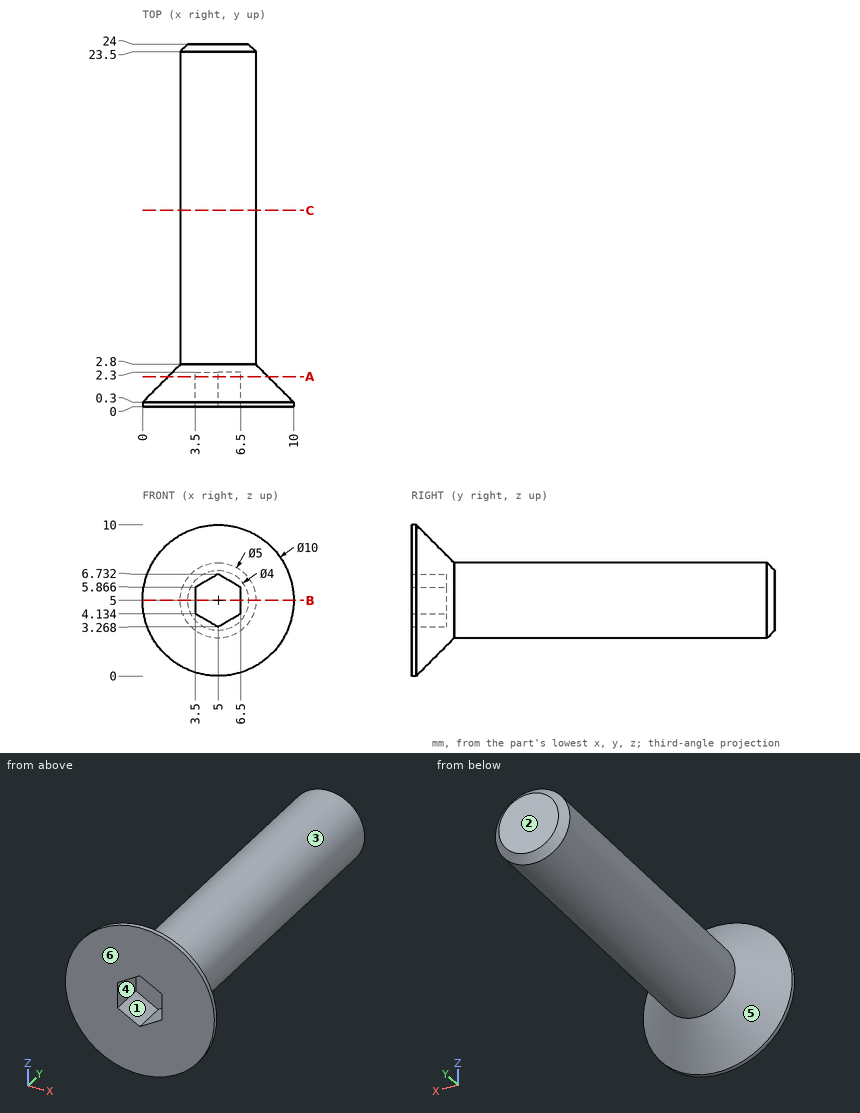
Input: dimensioned drawing with shaded views. Units: mm. Origin: part minimum x, y, z. A direction names the side the tool comes from. Coordinates: 2 decimals unless noted, no trailing zeros. Write each loop counter-clockwise with the first axis right and the second up, starting at its lowest first coordinate (ties: lowest second). Pieces come first, ordered by that corner, then holes. Notation, with made-up numbers: M -7,5.25 L 6,5.25 A17 ccw 6,9.25 Z; hole C 84,11.5 d4. An arc over 180 degrees is marked long. Answer as CSV lines item,"result". Start each with the question number.
Q1. Reachability of the marked faces 1, 2 and 3 from +Z, -Z, +X, -X, +Y, -Y: full face, straight path, thin tool, end or side. Return the list, or none.
Q2. Pin query (flat end, axial travel): P1, Ø1, axis at x = 6, y = 19, coming from the -Z side; P2, Ø0.5, axis at y = 1, z = 4.5, coming from the -X side; P3, Ø5, axis at x = 7, y = 11, coming from the -Z side. Return the tip coordinate at first contact, or that it passes through.
Q3. Cut plane A-A on y = 2. Return the cut outline in (x, z).
Q4. Cut plane B-B on z = 5. Return the cut outline in (x, y).
Q5. Line query: line 1 (Z direction, x = 3.5, y = 6); line 2 (Y direction, x = 6.25, z = 4.5); line 3 (Y direction, x = 0.5, z = 5). Output: solid intervals per line, ascending. Write a range as from..to.
Q6. Cut plane C-C on y = 13. Return the cut outline in (x, z).
Q7. Mould query, pull axis X, two halves, no side actions, for the marked faces 4, 5 and 6. Classes: released by +X, released by -X, zero draft, split by the parting line, or undercut.
Findings below:
1,face 1,"-Y"
1,face 2,"+Z, -Z, +X, -X, +Y"
1,face 3,"+Y"
2,P1,"stops at z = 2.55"
2,P2,"stops at x = 0.48"
2,P3,"stops at z = 2.5"
3,outline,"C 5,5 d6.6; hole M 3.5,4.13 L 5,3.27 L 6.5,4.13 L 6.5,5.87 L 5,6.73 L 3.5,5.87 Z"
4,outline,"M 0,0 L 3.5,0 L 3.5,2.3 L 6.5,2.3 L 6.5,0 L 10,0 L 10,0.3 L 7.5,2.8 L 7.5,23.5 L 7,24 L 3,24 L 2.5,23.5 L 2.5,2.8 L 0,0.3 Z"
5,line 1,"z = 3..7"
5,line 2,"y = 2.3..24"
5,line 3,"y = 0..0.8"
6,outline,"C 5,5 d5"
7,face 4,"undercut"
7,face 5,"split by the parting line"
7,face 6,"zero draft"
